For this review, use the dimensioned drawing (mm, ordinates from the lowest corner) and the shaded views. A direction names the side the tool comes from. Coordinates: 2 decimals unless noted, no trailing zeros. Order: outer loops, then holes, each group sorted by start corner. A loop starts at its lowest first (then second) coordinate and runs counter-clockwise, first axis right, second up. Notation, with made-up numbers: M 34,-26.75 L 51,-26.75 A33 ccw 51,10.25 Z; hole C 9.5,-3.75 d2. An arc over 180 degrees is marked long. Write each question's results on one line, items separated by ' | '.
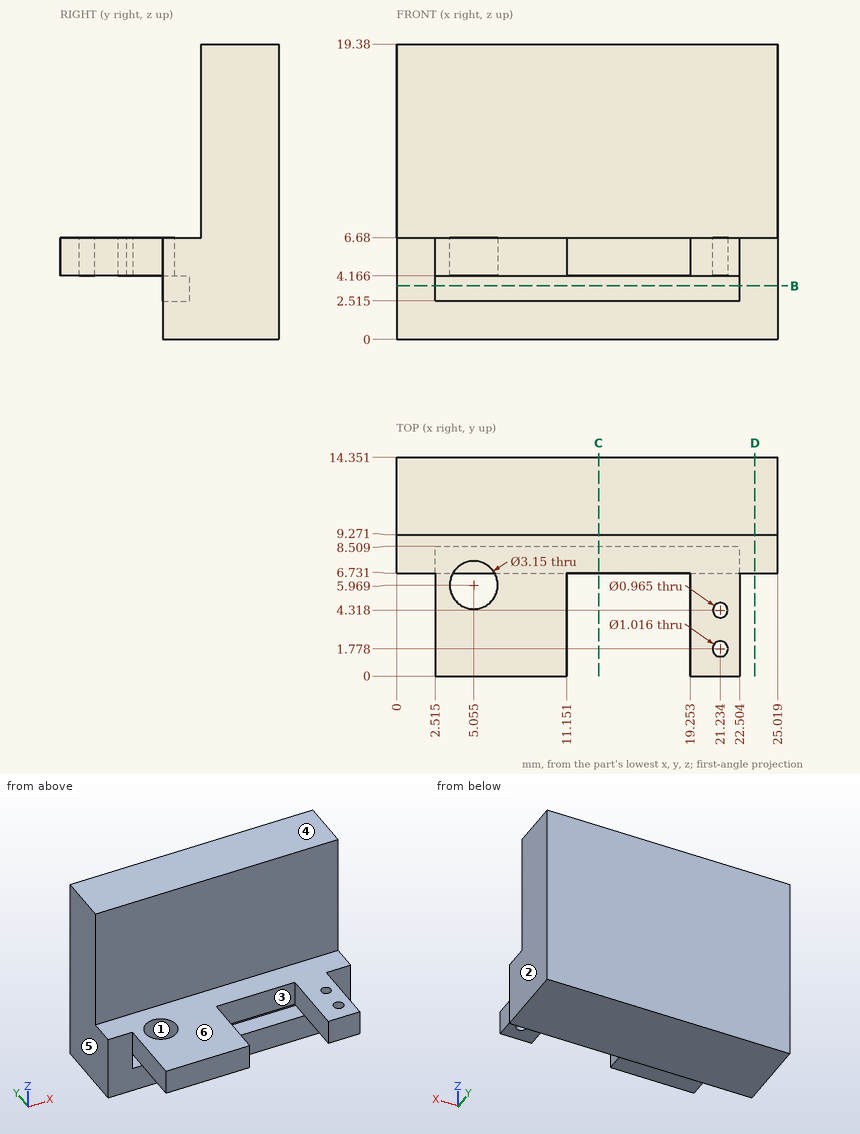
1) Take a section at C-C on x = 13.25. State the section outline as (y, z) points (1 decimal).
Solutions:
outline: M 6.7,0 L 14.4,0 L 14.4,19.4 L 9.3,19.4 L 9.3,6.7 L 6.7,6.7 L 6.7,4.2 L 8.5,4.2 L 8.5,2.5 L 6.7,2.5 Z
2) For the marked faces 5 and 6, list the 3-axis set-ups (+Z, -Z, +X, -X, +Y, -Y) from which the entire face can be reached by the end or side of a thin tool; tool diameter is ignored.
Solutions:
face 5: +Z, -Z, -X, +Y, -Y | face 6: +Z, +X, -X, -Y
3) Take a section at D-D on x = 23.5. State the section outline as (y, z) points, plus the area to 3 significant figures.
Solutions:
outline: M 6.73,0 L 14.35,0 L 14.35,19.38 L 9.27,19.38 L 9.27,6.68 L 6.73,6.68 Z | area: 115 mm2
4) Take a section at B-B on z = 3.5. State the section outline as (x, y) points (1 decimal), plus the area to 3 significant figures.
Solutions:
outline: M 0,6.7 L 2.5,6.7 L 2.5,8.5 L 22.5,8.5 L 22.5,6.7 L 25,6.7 L 25,14.4 L 0,14.4 Z | area: 155 mm2
5) For pin 1 (2 mm diameter, centred on y = 3.5, z = 5.5, fed in from -X) (1 decimal); pin 2 (10 mm diameter, centred on x = 18.5, z = 15, fed in from -Y); pin 3 (1.3 mm diameter, centred on y = 2.5, z = 6, fed in from +X), all flat-tipped, find the tip position at first contact; note any pin that passes through.
Solutions:
pin 1: x = 2.5 | pin 2: y = 9.27 | pin 3: x = 22.5
6) The part is to be moulded in two halves that separate along X. For the marked faces 1, 2, 3 and 4, say which applies: pulls with the +X half, pulls with the -X half, needs draft (parallel to the pull), parting line crosses it, or undercut.
Solutions:
face 1: undercut | face 2: pulls with the +X half | face 3: undercut | face 4: needs draft
7) To check wall thickness, follow line 1 along X through (y, z) = (8.25, 3.5) (1 decimal); line 2 along Y through (x, z) = (23, 4); line 3 along Y through (x, z) = (19.5, 14). State the ranges of each line that lie inside material, in increasing order.
Solutions:
line 1: 0 to 2.5, 22.5 to 25 | line 2: 6.73 to 14.35 | line 3: 9.27 to 14.35
